Can you work these out from the model? Positions are in its coordinate system, mm. Face numbers are marked on the shaded views. A direction names the side the tool comes from. Coordinates: 2 decimals unless noted, no trailing zeros. Order: outer loops, then holes, each group sorted by start corner. A loop starts at its lowest first (then second) coordinate and runs counter-clockwise, first axis right, second up. Notation, with made-up numbers: (67.25, 38.5) -> (101.25, 38.5) arc R13 ccw to (101.25, 43.5) -> close; hole circle Ø3 at (50.5, 80). An arc over 180 degrees is marked (long way). Answer as CSV lines item,"result".
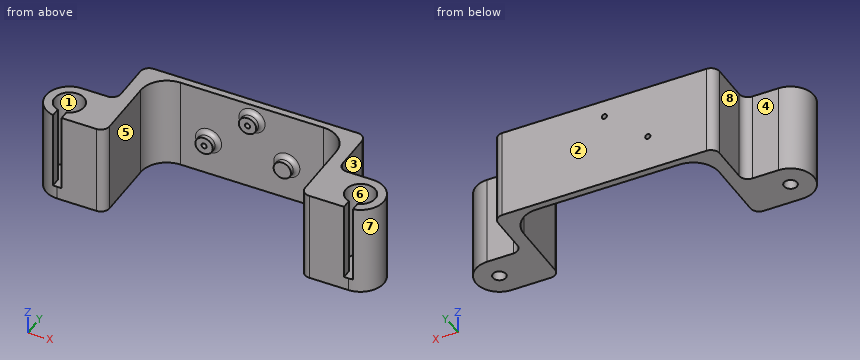
from build123d import *

# Parameters (mm, degrees)
SKETCH1_R           = 1.905
BOSS_EXTRUDE1_DEPTH = 26.67
CUT_EXTRUDE1_DEPTH  = 22.86
SKETCH8_W           = 57.15
SKETCH8_H           = 26.67
CUT_EXTRUDE4_DEPTH  = 1.778
SKETCH6_R           = 2.54
BOSS_EXTRUDE3_DEPTH = 2.54
SKETCH7_R           = 0.762
CUT_EXTRUDE3_DEPTH  = 7.62
FILLET1_R           = 2.54
FILLET4_R           = 7.62
SKETCH9_R           = 2.54
BOSS_EXTRUDE4_DEPTH = 2.54
FILLET3_R           = 1.27


with BuildPart() as part:
    # Sketch1 → Boss-Extrude1 (new body)
    with BuildSketch(Plane.XY):
        with BuildLine():
            Line((10.16, 22.86), (74.93, 22.86))
            Line((74.93, 22.86), (74.93, 6.858))
            Line((74.93, 6.858), (85.09, 6.858))
            ThreePointArc((85.09, 6.858), (91.948, 0), (85.09, -6.858))
            Line((85.09, -6.858), (71.12, -6.858))
            Line((71.12, -6.858), (71.12, -4.572))
            Line((71.12, -4.572), (71.12, 19.05))
            Line((71.12, 19.05), (42.545, 19.05))
            Line((42.545, 19.05), (13.97, 19.05))
            Line((13.97, 19.05), (13.97, -4.572))
            Line((13.97, -4.572), (13.97, -6.858))
            Line((13.97, -6.858), (0, -6.858))
            ThreePointArc((0, -6.858), (-6.858, 0), (0, 6.858))
            Line((0, 6.858), (10.16, 6.858))
            Line((10.16, 6.858), (10.16, 22.86))
        make_face()
        Circle(SKETCH1_R, mode=Mode.SUBTRACT)
        with Locations((85.09, 0)):
            Circle(SKETCH1_R, mode=Mode.SUBTRACT)
    extrude(amount=-BOSS_EXTRUDE1_DEPTH)

    # Sketch3 → Cut-Extrude1 (cut)
    with BuildSketch(Plane.XY):
        with BuildLine():
            Line((83.82, -4.12701151), (83.82, -6.858))
            Line((83.82, -6.858), (85.09, -6.858))
            ThreePointArc((85.09, -6.858), (85.727763736, -6.828281), (86.36, -6.739381574))
            Line((86.36, -6.739381574), (86.36, -4.12701151))
            ThreePointArc((86.36, -4.12701151), (85.09, 4.318), (83.82, -4.12701151))
        make_face()
        with BuildLine():
            Line((-1.27, -4.12701151), (-1.27, -6.739381574))
            ThreePointArc((-1.27, -6.739381574), (-0.637763736, -6.828281), (0, -6.858))
            Line((0, -6.858), (1.27, -6.858))
            Line((1.27, -6.858), (1.27, -4.12701151))
            ThreePointArc((1.27, -4.12701151), (0, 4.318), (-1.27, -4.12701151))
        make_face()
    extrude(amount=-CUT_EXTRUDE1_DEPTH, mode=Mode.SUBTRACT)

    # Sketch8 → Cut-Extrude4 (cut)
    with BuildSketch(Plane(origin=(0, 19.05, 0), x_dir=(-1, 0, 0), z_dir=(0, -1, 0))):
        with Locations((-42.545, 13.335)):
            Rectangle(SKETCH8_W, SKETCH8_H)
    extrude(amount=-CUT_EXTRUDE4_DEPTH, mode=Mode.SUBTRACT)

    # Sketch6 → Boss-Extrude3 (add)
    with BuildSketch(Plane(origin=(0, 20.828, 0), x_dir=(-1, 0, 0), z_dir=(0, -1, 0))):
        with Locations(Location((-42.545, 5.08, 0), (0, 0, 90))):
            Circle(SKETCH6_R)
        with Locations(Location((-29.845, 16.002, 0), (0, 0, 90))):
            Circle(SKETCH6_R)
    extrude(amount=BOSS_EXTRUDE3_DEPTH)

    # Sketch7 → Cut-Extrude3 (cut)
    with BuildSketch(Plane(origin=(0, 18.288, 0), x_dir=(-1, 0, 0), z_dir=(0, -1, 0))):
        with Locations(Location((-42.545, 5.08, 0), (0, 0, 90))):
            Circle(SKETCH7_R)
        with Locations(Location((-29.845, 16.002, 0), (0, 0, 90))):
            Circle(SKETCH7_R)
    extrude(amount=-CUT_EXTRUDE3_DEPTH, mode=Mode.SUBTRACT)

    # Fillet1
    fillet1_edges = [part.edges().sort_by_distance(p)[0] for p in [
        (10.16, 6.858, -13.335),
        (10.16, 22.86, -13.335),
        (74.93, 22.86, -13.335),
        (74.93, 6.858, -13.335),
        (71.12, -6.858, -13.335),
        (13.97, -6.858, -13.335),
    ]]
    fillet(fillet1_edges, radius=FILLET1_R)

    # Fillet4
    fillet4_edges = [part.edges().sort_by_distance(p)[0] for p in [
        (71.12, 20.828, -13.335),
        (13.97, 20.828, -13.335),
    ]]
    fillet(fillet4_edges, radius=FILLET4_R)

    # Sketch9 → Boss-Extrude4 (add)
    with BuildSketch(Plane(origin=(0, 20.828, 0), x_dir=(-1, 0, 0), z_dir=(0, -1, 0))):
        with Locations(Location((-52.705, 16.002, 0), (0, 0, 90))):
            Circle(SKETCH9_R)
    extrude(amount=BOSS_EXTRUDE4_DEPTH)

    # Fillet3
    fillet3_edges = [part.edges().sort_by_distance(p)[0] for p in [
        (42.545, 20.828, -2.54),
        (29.845, 20.828, -13.462),
        (52.705, 20.828, -13.462),
    ]]
    fillet(fillet3_edges, radius=FILLET3_R)


solid = part.part
Q1. For P1, Ø4, axis at x = 42.5, z = -6, coming from the -Y side; P2, Ø4.5, axis at x = 0, y = 0, coming from the +Z side; P3, Ø1.3, axis at y = -6, z = -7, coming from the -X side; P4, Ø3.5, axis at x = 85.09, y = 0, coming from the +Z side, each with a flat end and sliding along its axis, tell me the tip position at first contact or that it passes through.
Solution:
P1,"y = 18.29"
P2,"z = -22.86"
P3,"x = -4.29"
P4,"through"
Q2. Imagine slicing it at D-D (x = 79). List the corners of the cut face in (y, z) for me, and give its area (3 significant figures).
Solution:
outline,"(-6.86, -26.67) -> (6.86, -26.67) -> (6.86, 0) -> (-6.86, 0) -> close"
area,"366 mm2"
Q3. Imagine slicing it at C-C (y = 17.25). List the corners of the cut face in (x, z) for me.
Solution:
outline,"(10.16, -26.67) -> (15.13, -26.67) -> (15.13, 0) -> (10.16, 0) -> close; (69.96, -26.67) -> (74.93, -26.67) -> (74.93, 0) -> (69.96, 0) -> close"
Q4. We'd pull the mould along Y, two halves only. Please class the marked faces 6, 7 and 8: pulls with the +Y half, pulls with the -Y half, needs draft (parallel to the pull), parting line crosses it, or undercut.
Solution:
face 6,"undercut"
face 7,"parting line crosses it"
face 8,"needs draft"
Q5. If I drill on line 1 (X direction, y = 0, z = -14.5); line 2 (Y direction, x = 85.09, z = -24.4) (3 decimals); line 3 (X direction, y = 9.5, z = -6.25), over which ranges is the centre line in solid material (lowest first)?
Solution:
line 1,"-6.86 to -4.32, 4.32 to 13.97, 71.12 to 80.77, 89.41 to 91.95"
line 2,"-6.858 to -1.905, 1.905 to 6.858"
line 3,"10.16 to 13.97, 71.12 to 74.93"
Q6. Imagine slicing it at A-A (y = 0). List the corners of the cut face in (x, z) for me (3 decimals).
Solution:
outline,"(-6.858, -26.67) -> (-1.905, -26.67) -> (-1.905, -22.86) -> (-4.318, -22.86) -> (-4.318, 0) -> (-6.858, 0) -> close; (1.905, -26.67) -> (13.97, -26.67) -> (13.97, 0) -> (4.318, 0) -> (4.318, -22.86) -> (1.905, -22.86) -> close; (71.12, -26.67) -> (83.185, -26.67) -> (83.185, -22.86) -> (80.772, -22.86) -> (80.772, 0) -> (71.12, 0) -> close; (86.995, -26.67) -> (91.948, -26.67) -> (91.948, 0) -> (89.408, 0) -> (89.408, -22.86) -> (86.995, -22.86) -> close"
Q7. Which directions (+Z, -Z, +X, -X, +Y, -Y) give clear straight access to the entire face, cutting with the end or side of a thin tool? Please do the marked faces 1, 2, 3, 4 and 5.
Solution:
face 1,"+Z"
face 2,"+Z, -Z, +X, -X, +Y"
face 3,"+Z, -Z, +X, +Y"
face 4,"+Z, -Z, -X, +Y"
face 5,"+Z, -Z, -Y"
Q8. Imagine slicing it at B-B (z = -21). List the corners of the cut face in (x, y) for me, and give its area (3 significant figures).
Solution:
outline,"(-1.27, -6.74) -> (-1.27, -4.13) arc R4.32 cw (long way) to (1.27, -4.13) -> (1.27, -6.86) -> (11.43, -6.86) arc R2.54 ccw to (13.97, -4.32) -> (13.97, 13.21) arc R7.62 cw to (21.59, 20.83) -> (63.5, 20.83) arc R7.62 cw to (71.12, 13.21) -> (71.12, -4.32) arc R2.54 ccw to (73.66, -6.86) -> (83.82, -6.86) -> (83.82, -4.13) arc R4.32 cw (long way) to (86.36, -4.13) -> (86.36, -6.74) arc R6.86 ccw to (85.09, 6.86) -> (77.47, 6.86) arc R2.54 cw to (74.93, 9.4) -> (74.93, 20.32) arc R2.54 ccw to (72.39, 22.86) -> (12.7, 22.86) arc R2.54 ccw to (10.16, 20.32) -> (10.16, 9.4) arc R2.54 cw to (7.62, 6.86) -> (0, 6.86) arc R6.86 ccw to start"
area,"661 mm2"
